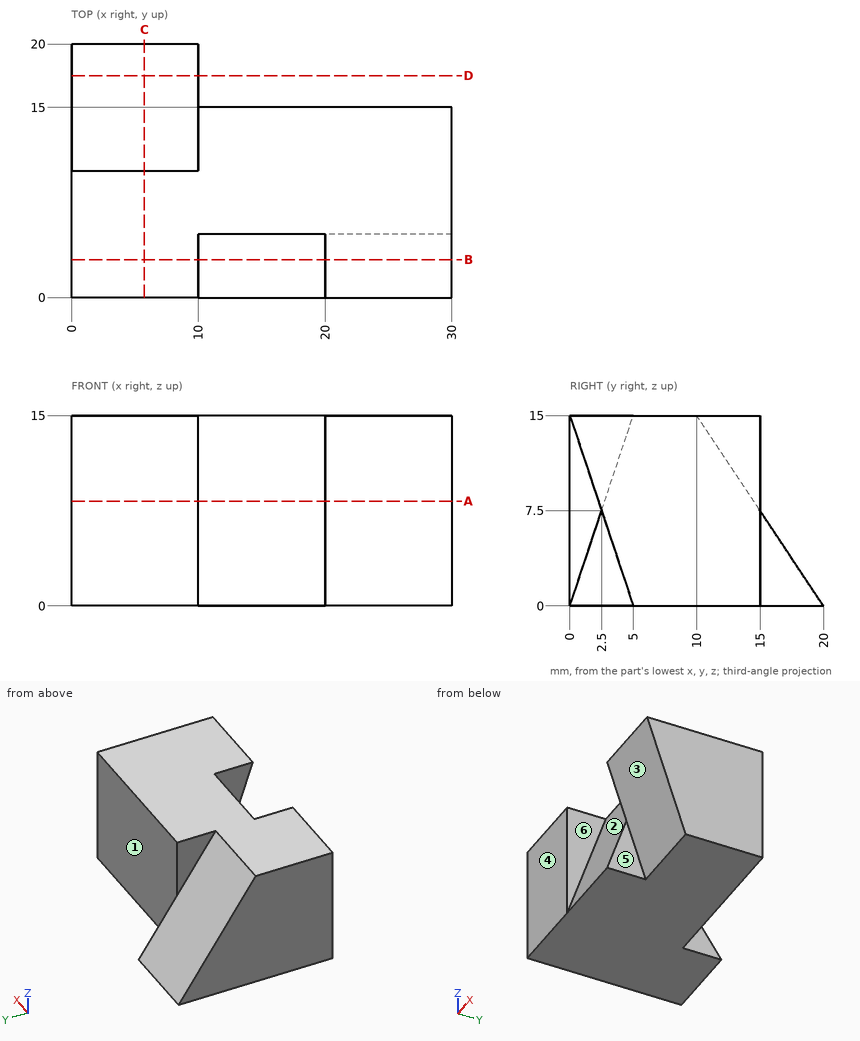
The drawing under review shows one solid part. Ordinate dimensions are in mm from its lowest x, y, z. A direction names the side the tool comes from. Round coordinates to 2 decimals unless told otherwise and drop trailing zeros. Order: outer loops, then holes, each group sorted by start corner. A loop starts at its lowest first (then second) coordinate and runs counter-clockwise, first axis right, second up. Notation, with made-up numbers: (15.25, 15.5) -> (30.25, 15.5) arc R27 ccw to (30.25, 32.5) -> close; hole circle Ø9 at (4, 1). An arc over 180 degrees is marked (long way). Return JSON: item names as keys, results as strings.
1. Take a section at D-D (y = 17.5). Write out the cut boundary in (x, z), then the cut area to 3 significant figures.
Answer block:
{"outline": "(0, 0) -> (10, 0) -> (10, 3.75) -> (0, 3.75) -> close", "area": "37.5 mm²"}
2. Take a section at A-A (z = 8.25). Write out the cut boundary in (x, y), then the cut area to 3 significant figures.
Answer block:
{"outline": "(0, 0) -> (10, 0) -> (10, 2.75) -> (20, 2.75) -> (20, 2.25) -> (30, 2.25) -> (30, 15) -> (10, 15) -> (10, 14.5) -> (0, 14.5) -> close", "area": "395 mm²"}
3. Take a section at B-B (y = 3). Write out the cut boundary in (x, z).
Answer block:
{"outline": "(0, 0) -> (20, 0) -> (20, 6) -> (30, 6) -> (30, 15) -> (20, 15) -> (20, 9) -> (10, 9) -> (10, 15) -> (0, 15) -> close"}
4. Insertion check: P1, Ø4.5, axis at x = 22, z = 10.5, coming from the +Y side; P2, Ø3, axis at x = 27, z = 6.5, coming from the -Y side. Each pin has a flat end and moves straight along its axis. Give the tip position at first contact, or say it passes through.
Answer block:
{"P1": "stops at y = 15", "P2": "stops at y = 2.33"}
5. Take a section at C-C (x = 5.75). Write out the cut boundary in (y, z), then the cut area to 3 significant figures.
Answer block:
{"outline": "(0, 0) -> (20, 0) -> (10, 15) -> (0, 15) -> close", "area": "225 mm²"}
6. The part is to be moulded in two halves that separate along X. For the marked faces 4, 5 and 6, say which applies: +X half, -X half, draft (parallel to the pull), parting line (faces both ways), or undercut.
Answer block:
{"face 4": "draft", "face 5": "+X half", "face 6": "undercut"}
7. For the marked faces 1, 2 and 3, list the 3-axis set-ups (+Z, -Z, +X, -X, +Y, -Y) from which the entire face can be reached by the end or side of a thin tool; tool diameter is ignored.
Answer block:
{"face 1": "+Z, -Z, +X, +Y", "face 2": "+Z, -Y", "face 3": "-Z, +X, -Y"}
8. For L1, parallel to X at y = 2, z = 11.5; L2, parallel to X at y = 15.75, z = 5.25; L3, parallel to X at y = 2.25, z = 5.5, list the stretches that pass through material, from the lowest coordinate up. Write a range as [from, to].
Answer block:
{"L1": "x = [0, 10], [20, 30]", "L2": "x = [0, 10]", "L3": "x = [0, 20]"}
